Geometry: final body of the model. Coordinates: model frame, mm. A direction names the side the tool comes from. Give positions to 0.01 mm unless a question says otherwise; leave off trailing zeros. Loops run counter-clockwise (first coordinate to the right, second up) from the corner with the lowest first, then second, coordinate; pieces in that order, holes last. Notation, with made-up numbers: (-27.5, 12.5) - (24.5, 12.5) arc R14 cw to (24.5, 36.5) - close; hole circle Ø9 at (50, 17.5). An arc over 180 degrees is marked (long way). Use one line per item in the form item = value.
```python
from build123d import *

# Parameters (mm, degrees)
SKETCH_1_W      = 50
SKETCH_1_H      = 10
EXTRUDE_1_DEPTH = 120
EXTRUDE_2_DEPTH = 10
SKETCH_2_R      = 5
EXTRUDE_3_DEPTH = 50


with BuildPart() as part:
    # 草图1 → 凸台-拉伸1 (new body)
    with BuildSketch(Plane.XY):
        Rectangle(SKETCH_1_W, SKETCH_1_H)
    extrude(amount=EXTRUDE_1_DEPTH)

    # 草图3 → 凸台-拉伸2 (add)
    with BuildSketch(Plane.XY.offset(120)):
        with BuildLine():
            Line((-50, -55), (-46, -55))
            ThreePointArc((-46, -55), (0, -9), (46, -55))
            Line((46, -55), (50, -55))
            ThreePointArc((50, -55), (43.301270189, -30), (25, -11.698729811))
            Line((25, -11.698729811), (25, -5))
            Line((25, -5), (-25, -5))
            Line((-25, -5), (-25, -11.698729811))
            ThreePointArc((-25, -11.698729811), (-43.301270189, -30), (-50, -55))
        make_face()
    extrude(amount=-EXTRUDE_2_DEPTH)

    # 草图2 → 凸台-拉伸3 (add)
    with BuildSketch(Plane(origin=(25, 0, 0), x_dir=(0, 0, -1), z_dir=(1, 0, 0))):
        Circle(SKETCH_2_R)
    extrude(amount=-EXTRUDE_3_DEPTH)


solid = part.part
```
(1) Cut plane A-A (y = -45). Return the cut outline in (x, z).
Solution:
outline = (-48.99, 110) - (-44.9, 110) - (-44.9, 120) - (-48.99, 120) - close; (44.9, 110) - (48.99, 110) - (48.99, 120) - (44.9, 120) - close
(2) Access query for faces 1 (the face through (25, 0, 58)), 2 (the face through (0, -8, 110)), 3 (the face through (48, -55, 115)), 4 (the face through (-25, 0, 58)). Directions: +Z, -Z, +X, -X, +Y, -Y. A direction counts if a zero-diameter tool reaches every point of the face in a straight line with its end or side. Return the directions, or none.
Solution:
face_1 = +Z, -Z, +X, +Y
face_2 = -Z, +X, -X, -Y
face_3 = +Z, -Z, +X, -X, -Y
face_4 = +Z, -Z, -X, +Y
(3) Material intervals for L1, parallel to Y at x = -13, z = 19.5; L2, parallel to X at y = -3, z = 56.5, sorted ascending. Write a range as from..to.
Solution:
L1 = -5..5
L2 = -25..25
(4) Cut plane C-C (z = 95.5). Return the cut outline in (x, y), plus the area to 3 significant figures.
Solution:
outline = (-25, -5) - (25, -5) - (25, 5) - (-25, 5) - close
area = 500 mm2
(5) Pin query (flat end, axial travel): P1, Ø8.5, axis at y = -3, z = 87, coming from the +X side; P2, Ø8.5, axis at y = 0.5, z = 84, coming from the -X side. Return the tip coordinate at first contact, or that it passes through.
Solution:
P1 = 25
P2 = -25
(6) Cut plane B-B (x = 0). Return the cut outline in (y, z).
Solution:
outline = (-9, 110) - (-5, 110) - (-5, 0) arc R5 ccw to (5, 0) - (5, 120) - (-9, 120) - close
(7) Cut plane D-D (y = -18). Return the cut outline in (x, z).
Solution:
outline = (-33.63, 110) - (-27.33, 110) - (-27.33, 120) - (-33.63, 120) - close; (27.33, 110) - (33.63, 110) - (33.63, 120) - (27.33, 120) - close
